Geometry check sheet. Reference: drawing and pictorial views, mm from the part's lowest x, y, z. A direction names the side the tool comes from. Round coordinates to 2 decimals unless told otherwise and drop trailing zeros. Write each loop counter-clockwise with the first axis right and the second up, starting at its lowest first coordinate (ties: lowest second). Pieces come first, ordered by that corner, then holes.
Item 1: Section check D-D, the plane x = 17. Record the cut outline in (y, z), plus the area to 3 significant figures.
Item 2: Depth check by flat-ended pin: pin 1 (8 mm diameter, centred on y = 13, z = 60.5, fed in from +X); pin 2 (11.5 mm diameter, centred on x = 30, y = 11.5, fed in from +Z); pin 3 (4.5 mm diameter, centred on x = 21.5, z = 59, fed in from +Y); pin 4 (1.5 mm diameter, centred on x = 7, y = 30, fed in from -Z). Enter the tip coordinate at first touch or a pass-through.
Item 3: Section check A-A, the plane y = 11.5. Record the cut outline in (x, z) (1 decimal).
Item 4: Set-up check for the marked faces 1, 2 and 3: record each of +Z, -Z, +X, -X, +Y, -Y from which the full face is reachable in a straight line by a thin tool's end or side.
Item 5: Material ranges on line 1 along Z through (x, y) = (30.5, 20); line 2 along X through (y, z) = (7.5, 41); line 3 along Y through (x, z) = (30, 3), recorded low to high.
Item 6: Section check C-C, the plane z = 97.5. Record the cut outline in (x, y), plus the area to 3 significant figures.
Item 7: Release check for a two-part mould opening along Z. For the marked faces 4, 5 and 6 record: pulls with the +Z half, pulls with the -Z half, needs draft (parallel to the pull), parting line crosses it, or undercut.
Item 8: Section check B-B, the plane x = 30. Record the cut outline in (y, z), plus the area to 3 significant figures.
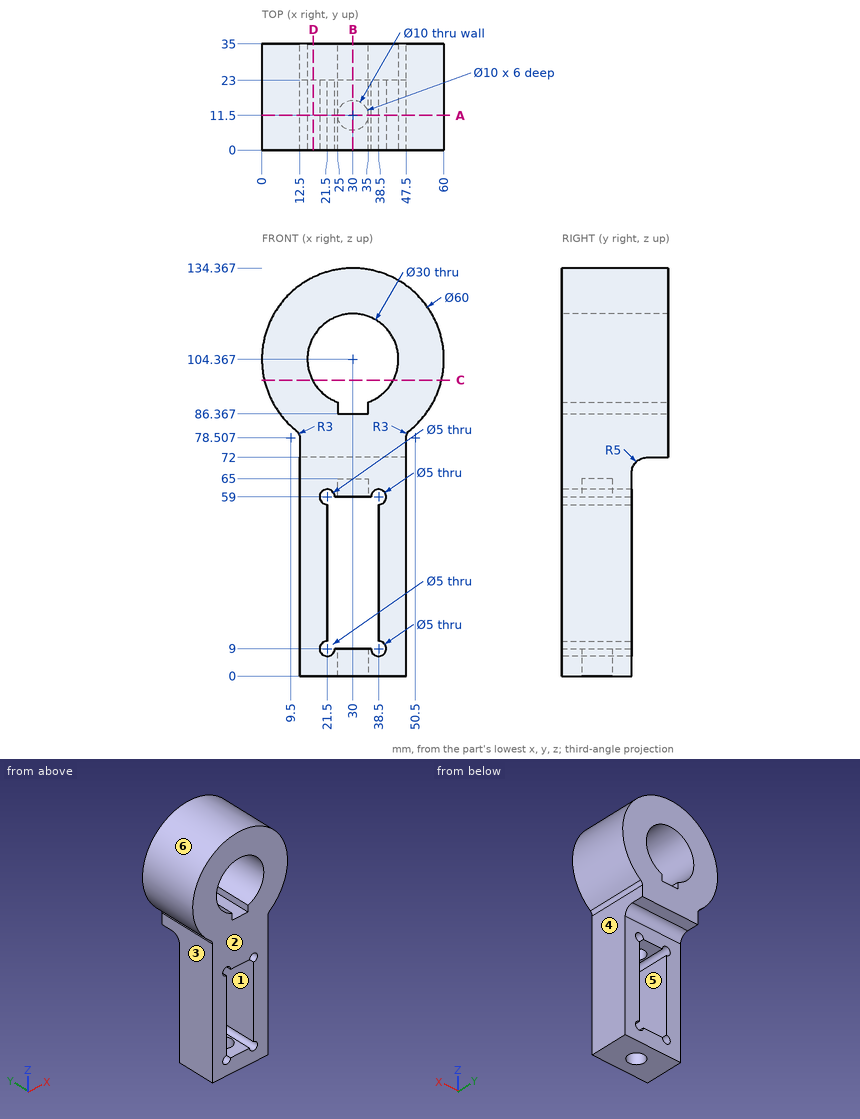
Values found:
1. outline: (0, 0) - (23, 0) - (23, 67) arc R5 cw to (28, 72) - (35, 72) - (35, 96.88) - (0, 96.88) - close; (0, 111.85) - (35, 111.85) - (35, 131.4) - (0, 131.4) - close
1. area: 3,220 mm2
2. pin 1: stops at x = 47.5
2. pin 2: stops at z = 134.37
2. pin 3: passes through
2. pin 4: stops at z = 84.24
3. outline: (11.4, 80.9) arc R3 cw to (12.5, 78.5) - (12.5, 0) - (25, 0) - (25, 9) - (24, 9) arc R2.5 cw (long way) to (21.5, 11.5) - (21.5, 56.5) arc R2.5 cw (long way) to (24, 59) - (25, 59) - (25, 65) - (35, 65) - (35, 59) - (36, 59) arc R2.5 cw (long way) to (38.5, 56.5) - (38.5, 11.5) arc R2.5 cw (long way) to (36, 9) - (35, 9) - (35, 0) - (47.5, 0) - (47.5, 78.5) arc R3 cw to (48.6, 80.9) arc R30 ccw (long way) to start; hole (25, 86.4) - (35, 86.4) - (35, 90.2) arc R15 ccw (long way) to (25, 90.2) - close
4. face 1: +Y, -Y
4. face 2: +Z, -Z, +X, -X, -Y
4. face 3: -Z, -X, +Y, -Y
5. line 1: z = 0 to 9, 59 to 86.37, 119.36 to 134.36
5. line 2: x = 12.5 to 21.5, 38.5 to 47.5
5. line 3: y = 0 to 6.5, 16.5 to 23
6. outline: (0.8, 0) - (16.66, 0) - (16.66, 35) - (0.8, 35) - close; (43.34, 0) - (59.2, 0) - (59.2, 35) - (43.34, 35) - close
6. area: 1,110 mm2
7. face 4: needs draft
7. face 5: undercut
7. face 6: parting line crosses it
8. outline: (0, 0) - (6.5, 0) - (6.5, 9) - (0, 9) - close; (0, 59) - (6.5, 59) - (6.5, 65) - (16.5, 65) - (16.5, 59) - (23, 59) - (23, 67) arc R5 cw to (28, 72) - (35, 72) - (35, 86.37) - (0, 86.37) - close; (0, 119.37) - (35, 119.37) - (35, 134.37) - (0, 134.37) - close; (16.5, 0) - (23, 0) - (23, 9) - (16.5, 9) - close
8. area: 1,390 mm2
